The model under review builds one solid part; all positions refer to its coordinate system, in mm. A direction names the side the tool comes from. Give positions to 0.01 mm unless a question says otherwise; leave off trailing zeros. Loops run counter-clockwise (first coordinate to the right, second up) from the corner with the lowest first, then second, coordinate; pieces in that order, holes last. Notation, with made-up numbers: M 58,-17.75 L 99,-17.75 A15 ccw 99,-3.75 Z; hole C 14.5,60.25 d6. An arc over 180 degrees is marked long. One line per item, written item: value. Start each with the question number.
Q1. For pin 1 (0.5 mm diameter, centred on x = 3, z = -62, fed in from -Y); pin 2 (2.5 mm diameter, centred on x = 3.5, y = -45, fed in from +Z), all flat-tipped, find the tip position at first contact; note any pin that passes through.
Q2. We need section D-D on y = -43.5. Write out the cut boundary in (x, z).
Q3. We need section C-C on x = 2.75. Write out the cut boundary in (y, z), plus the area to 3 significant figures.
Q4. We need section A-A on y = -9. Write out the cut boundary in (x, z), plus the area to 3 significant figures.
Q5. Mouldability with a two-part tool opening along Z and no side actions: class faces 4 (the face through (2.47, -19.92, -9.26)), 5 (the face through (2, -20, 24.3)), 6 (the face through (2, -49.188, -19)) as released by +Z, released by -Z, zero draft, split by the parting line, or undercut.
Q6. To check wall thickness, follow line 1 along Z through (x, y) = (3.8, -31); line 2 along Z through (x, y) = (4.4, -29.5); line 3 along Z through (x, y) = (4.8, -46). State the ranges of each line that lie inside material, in increasing order. Write a range as from..to.
Q7. We need section B-B on z = -34. Write out the cut boundary in (x, y), plus the area to 3 significant figures.
Q8. For faces 1 (the face through (2, -45, -61.251)), 2 (the face through (2, 0, -20)), 3 (the face through (2, -45, 23.592)), list the 3-axis set-ups (+Z, -Z, +X, -X, +Y, -Y) from which the entire face can be reached by the end or side of a thin tool; tool diameter is ignored.
```python
from build123d import *

# Parameters (mm, degrees)
F0_W     = 40.193792
F0_H     = 87.127595
F1_DEPTH = 5
F3_D     = 30
F4_W     = 10.118723
F4_H     = 84.843202
F5_DEPTH = 5


with BuildPart() as f1:
    # F0 (on Right) → F1 (new body)
    with BuildSketch(Plane.YZ):
        with Locations((-20.096896, -19.263864)):
            Rectangle(F0_W, F0_H)
    extrude(amount=F1_DEPTH)

    # F3 (through all)
    with Locations(Plane.YZ.offset(5)):
        with Locations((-21.870809, -24.133997)):
            Hole(F3_D / 2)

    # F4 (on Right) → F5 (join)
    with BuildSketch(Plane.YZ):
        with Locations((-44.12885, -18.829883)):
            Rectangle(F4_W, F4_H)
    extrude(amount=F5_DEPTH)


solid = f1.part
```
Solved:
1. pin 1: y = -40.19
1. pin 2: z = 23.59
2. outline: M 0,-61.25 L 5,-61.25 L 5,23.59 L 0,23.59 Z
3. outline: M -49.19,-61.25 L -40.19,-61.25 L -40.19,-62.83 L 0,-62.83 L 0,24.3 L -40.19,24.3 L -40.19,23.59 L -49.19,23.59 Z; hole C -21.87,-24.13 d30
3. area: 3,560 mm2
4. outline: M 0,-62.83 L 5,-62.83 L 5,-31.84 L 0,-31.84 Z; M 0,-16.43 L 5,-16.43 L 5,24.3 L 0,24.3 Z
4. area: 359 mm2
5. face 4: undercut
5. face 5: released by +Z
5. face 6: zero draft
6. line 1: -62.83..-36.04, -12.23..24.3
6. line 2: -62.83..-37.05, -11.22..24.3
6. line 3: -61.25..23.59
7. outline: M 0,-49.19 L 5,-49.19 L 5,-33.17 L 0,-33.17 Z; M 0,-10.57 L 5,-10.57 L 5,0 L 0,0 Z
7. area: 133 mm2
8. face 1: -Z, +X, -X, -Y
8. face 2: +Z, -Z, +X, -X, +Y
8. face 3: +Z, +X, -X, -Y
